For this review, use the dimensioned drawing (mm, ordinates from the lowest corner) and the shaded views. Coordinates: 2 decimals unless noted, no trailing zeros. Loops run counter-clockwise (first coordinate to the right, second up) from the corner with the lowest first, then second, coordinate; pieces in that order, holes last. Notation, with made-up numbers: (44.5, 26.25) -> (83.5, 26.25) arc R6 ccw to (83.5, 30.25) -> close; hole circle Ø1 at (-2.75, 81.5). An arc over 180 degrees is marked (long way). Answer as a JSON object with one key per item and string values.
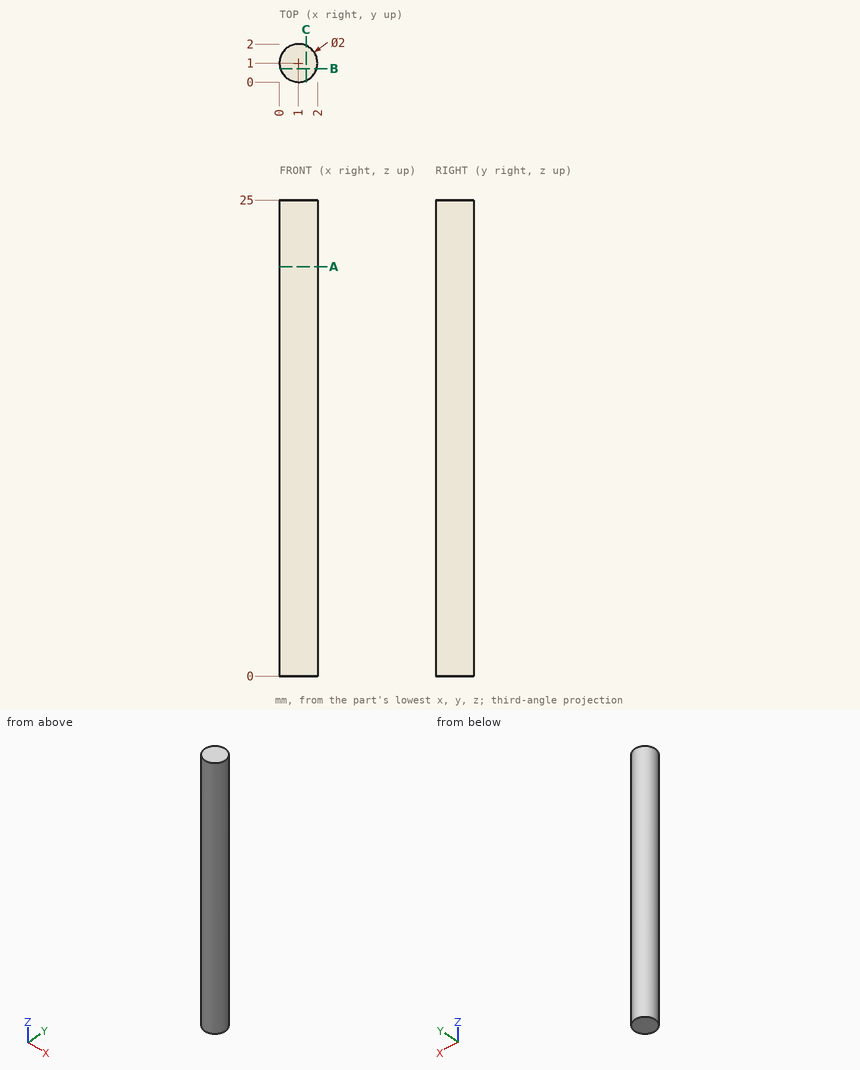
1) Add section C-C, the plane x = 1.4. Give the boundary of the cut face in (y, z).
Completed:
{"outline": "(0.08, 0) -> (1.92, 0) -> (1.92, 25) -> (0.08, 25) -> close"}
2) Wall thickness on probe 1 along X at (y, z) = (1.1, 21.75); probe 2 along X at (y, z) = (1.4, 16): over which ranges is each line inside the solid? List them lowest first.
Completed:
{"probe 1": "0.01 to 1.99", "probe 2": "0.08 to 1.92"}
3) Add section A-A, the plane z = 21.5. Give the boundary of the cut face in (x, y), and give its area (3 significant figures).
Completed:
{"outline": "circle Ø2 at (1, 1)", "area": "3.14 mm²"}
4) Add section B-B, the plane y = 0.7. Give the boundary of the cut face in (x, z), and give its area (3 significant figures).
Completed:
{"outline": "(0.05, 0) -> (1.95, 0) -> (1.95, 25) -> (0.05, 25) -> close", "area": "47.7 mm²"}
